```python
from build123d import *

# Parameters (mm, degrees)
CROQUIS1_R              = 2.1
CROQUIS1_R_2            = 3.4
SALIENTE_EXTRUIR1_DEPTH = 400


with BuildPart() as part:
    # Croquis1 → Saliente-Extruir1 (new body)
    with BuildSketch(Plane(origin=(0, 0, -50), x_dir=(-1, 0, 0), z_dir=(0, 0, -1))):
        with BuildLine():
            Line((14.7, -5.1), (14.3, -5.1))
            ThreePointArc((14.3, -5.1), (14.087867966, -5.012132034), (14, -4.8))
            Line((14, -4.8), (14, -4.4))
            ThreePointArc((14, -4.4), (13.912132034, -4.187867966), (13.7, -4.1))
            Line((13.7, -4.1), (13.3, -4.1))
            ThreePointArc((13.3, -4.1), (13.087867966, -4.187867966), (13, -4.4))
            Line((13, -4.4), (13, -7.95))
            ThreePointArc((13, -7.95), (12.912132034, -8.162132034), (12.7, -8.25))
            Line((12.7, -8.25), (9.789264108, -8.25))
            ThreePointArc((9.789264108, -8.25), (9.674477865, -8.22717164), (9.577160832, -8.162160788))
            Line((9.577160832, -8.162160788), (5.887896723, -4.473896751))
            ThreePointArc((5.887896723, -4.473896751), (5.822843922, -4.376559778), (5.8, -4.261735963))
            Line((5.8, -4.261735963), (5.8, 4.260735931))
            ThreePointArc((5.8, 4.260735931), (5.82283614, 4.375540961), (5.887867966, 4.472867966))
            Line((5.887867966, 4.472867966), (9.577132034, 8.162132034))
            ThreePointArc((9.577132034, 8.162132034), (9.674459039, 8.22716386), (9.789264069, 8.25))
            Line((9.789264069, 8.25), (12.7, 8.25))
            ThreePointArc((12.7, 8.25), (12.912132034, 8.162132034), (13, 7.95))
            Line((13, 7.95), (13, 4.4))
            ThreePointArc((13, 4.4), (13.087867966, 4.187867966), (13.3, 4.1))
            Line((13.3, 4.1), (13.7, 4.1))
            ThreePointArc((13.7, 4.1), (13.912132034, 4.187867966), (14, 4.4))
            Line((14, 4.4), (14, 4.8))
            ThreePointArc((14, 4.8), (14.087867966, 5.012132034), (14.3, 5.1))
            Line((14.3, 5.1), (14.7, 5.1))
            ThreePointArc((14.7, 5.1), (14.912132034, 5.187867966), (15, 5.4))
            Line((15, 5.4), (15, 12.5))
            ThreePointArc((15, 12.5), (14.267766953, 14.267766953), (12.5, 15))
            Line((12.5, 15), (5.4, 15))
            ThreePointArc((5.4, 15), (5.187867966, 14.912132034), (5.1, 14.7))
            Line((5.1, 14.7), (5.1, 14.3))
            ThreePointArc((5.1, 14.3), (5.012132034, 14.087867966), (4.8, 14))
            Line((4.8, 14), (4.4, 14))
            ThreePointArc((4.4, 14), (4.187867966, 13.912132034), (4.1, 13.7))
            Line((4.1, 13.7), (4.1, 13.3))
            ThreePointArc((4.1, 13.3), (4.187867966, 13.087867966), (4.4, 13))
            Line((4.4, 13), (7.95, 13))
            ThreePointArc((7.95, 13), (8.162132034, 12.912132034), (8.25, 12.7))
            Line((8.25, 12.7), (8.25, 9.788264069))
            ThreePointArc((8.25, 9.788264069), (8.22716386, 9.673459039), (8.162132034, 9.576132034))
            Line((8.162132034, 9.576132034), (4.473867966, 5.887867966))
            ThreePointArc((4.473867966, 5.887867966), (4.376540961, 5.82283614), (4.261735931, 5.8))
            Line((4.261735931, 5.8), (-4.260735892, 5.8))
            ThreePointArc((-4.260735892, 5.8), (-4.375522135, 5.82282836), (-4.472839168, 5.887839212))
            Line((-4.472839168, 5.887839212), (-8.162103277, 9.576103249))
            ThreePointArc((-8.162103277, 9.576103249), (-8.227156078, 9.673440222), (-8.25, 9.788264037))
            Line((-8.25, 9.788264037), (-8.25, 12.7))
            ThreePointArc((-8.25, 12.7), (-8.162132034, 12.912132034), (-7.95, 13))
            Line((-7.95, 13), (-4.4, 13))
            ThreePointArc((-4.4, 13), (-4.187867966, 13.087867966), (-4.1, 13.3))
            Line((-4.1, 13.3), (-4.1, 13.7))
            ThreePointArc((-4.1, 13.7), (-4.187867966, 13.912132034), (-4.4, 14))
            Line((-4.4, 14), (-4.8, 14))
            ThreePointArc((-4.8, 14), (-5.012132034, 14.087867966), (-5.1, 14.3))
            Line((-5.1, 14.3), (-5.1, 14.7))
            ThreePointArc((-5.1, 14.7), (-5.187867966, 14.912132034), (-5.4, 15))
            Line((-5.4, 15), (-12.5, 15))
            ThreePointArc((-12.5, 15), (-14.267766953, 14.267766953), (-15, 12.5))
            Line((-15, 12.5), (-15, 5.4))
            ThreePointArc((-15, 5.4), (-14.912132034, 5.187867966), (-14.7, 5.1))
            Line((-14.7, 5.1), (-14.3, 5.1))
            ThreePointArc((-14.3, 5.1), (-14.087867966, 5.012132034), (-14, 4.8))
            Line((-14, 4.8), (-14, 4.4))
            ThreePointArc((-14, 4.4), (-13.912132034, 4.187867966), (-13.7, 4.1))
            Line((-13.7, 4.1), (-13.3, 4.1))
            ThreePointArc((-13.3, 4.1), (-13.087867966, 4.187867966), (-13, 4.4))
            Line((-13, 4.4), (-13, 7.95))
            ThreePointArc((-13, 7.95), (-12.912132034, 8.162132034), (-12.7, 8.25))
            Line((-12.7, 8.25), (-9.788264037, 8.25))
            ThreePointArc((-9.788264037, 8.25), (-9.673440222, 8.227156078), (-9.576103249, 8.162103277))
            Line((-9.576103249, 8.162103277), (-5.887839212, 4.472839168))
            ThreePointArc((-5.887839212, 4.472839168), (-5.82282836, 4.375522135), (-5.8, 4.260735892))
            Line((-5.8, 4.260735892), (-5.8, -4.261735931))
            ThreePointArc((-5.8, -4.261735931), (-5.82283614, -4.376540961), (-5.887867966, -4.473867966))
            Line((-5.887867966, -4.473867966), (-9.576132034, -8.162132034))
            ThreePointArc((-9.576132034, -8.162132034), (-9.673459039, -8.22716386), (-9.788264069, -8.25))
            Line((-9.788264069, -8.25), (-12.7, -8.25))
            ThreePointArc((-12.7, -8.25), (-12.912132034, -8.162132034), (-13, -7.95))
            Line((-13, -7.95), (-13, -4.4))
            ThreePointArc((-13, -4.4), (-13.087867966, -4.187867966), (-13.3, -4.1))
            Line((-13.3, -4.1), (-13.7, -4.1))
            ThreePointArc((-13.7, -4.1), (-13.912132034, -4.187867966), (-14, -4.4))
            Line((-14, -4.4), (-14, -4.8))
            ThreePointArc((-14, -4.8), (-14.087867966, -5.012132034), (-14.3, -5.1))
            Line((-14.3, -5.1), (-14.7, -5.1))
            ThreePointArc((-14.7, -5.1), (-14.912132034, -5.187867966), (-15, -5.4))
            Line((-15, -5.4), (-15, -12.5))
            ThreePointArc((-15, -12.5), (-14.267766953, -14.267766953), (-12.5, -15))
            Line((-12.5, -15), (-5.4, -15))
            ThreePointArc((-5.4, -15), (-5.187867966, -14.912132034), (-5.1, -14.7))
            Line((-5.1, -14.7), (-5.1, -14.3))
            ThreePointArc((-5.1, -14.3), (-5.012132034, -14.087867966), (-4.8, -14))
            Line((-4.8, -14), (-4.4, -14))
            ThreePointArc((-4.4, -14), (-4.187867966, -13.912132034), (-4.1, -13.7))
            Line((-4.1, -13.7), (-4.1, -13.3))
            ThreePointArc((-4.1, -13.3), (-4.187867966, -13.087867966), (-4.4, -13))
            Line((-4.4, -13), (-7.95, -13))
            ThreePointArc((-7.95, -13), (-8.162132034, -12.912132034), (-8.25, -12.7))
            Line((-8.25, -12.7), (-8.25, -9.789264069))
            ThreePointArc((-8.25, -9.789264069), (-8.22716386, -9.674459039), (-8.162132034, -9.577132034))
            Line((-8.162132034, -9.577132034), (-4.472867966, -5.887867966))
            ThreePointArc((-4.472867966, -5.887867966), (-4.375540961, -5.82283614), (-4.260735931, -5.8))
            Line((-4.260735931, -5.8), (4.261735963, -5.8))
            ThreePointArc((4.261735963, -5.8), (4.376559778, -5.822843922), (4.473896751, -5.887896723))
            Line((4.473896751, -5.887896723), (8.162160788, -9.577160832))
            ThreePointArc((8.162160788, -9.577160832), (8.22717164, -9.674477865), (8.25, -9.789264108))
            Line((8.25, -9.789264108), (8.25, -12.7))
            ThreePointArc((8.25, -12.7), (8.162132034, -12.912132034), (7.95, -13))
            Line((7.95, -13), (4.4, -13))
            ThreePointArc((4.4, -13), (4.187867966, -13.087867966), (4.1, -13.3))
            Line((4.1, -13.3), (4.1, -13.7))
            ThreePointArc((4.1, -13.7), (4.187867966, -13.912132034), (4.4, -14))
            Line((4.4, -14), (4.8, -14))
            ThreePointArc((4.8, -14), (5.012132034, -14.087867966), (5.1, -14.3))
            Line((5.1, -14.3), (5.1, -14.7))
            ThreePointArc((5.1, -14.7), (5.187867966, -14.912132034), (5.4, -15))
            Line((5.4, -15), (12.5, -15))
            ThreePointArc((12.5, -15), (14.267766953, -14.267766953), (15, -12.5))
            Line((15, -12.5), (15, -5.4))
            ThreePointArc((15, -5.4), (14.912132034, -5.187867966), (14.7, -5.1))
        make_face()
        with Locations((-11.7, 11.7)):
            Circle(CROQUIS1_R, mode=Mode.SUBTRACT)
        with Locations((-11.7, -11.7)):
            Circle(CROQUIS1_R, mode=Mode.SUBTRACT)
        Circle(CROQUIS1_R_2, mode=Mode.SUBTRACT)
        with Locations((11.7, 11.7)):
            Circle(CROQUIS1_R, mode=Mode.SUBTRACT)
        with Locations((11.7, -11.7)):
            Circle(CROQUIS1_R, mode=Mode.SUBTRACT)
    extrude(amount=-SALIENTE_EXTRUIR1_DEPTH)


solid = part.part
```
The listing builds one solid part. Answer for the finished solid, in the listing's coordinates (mm). Round coordinates to 2 decimals unless told otherwise and drop trailing zeros. Order: outer loops, then holes, each group sorted by start corner. A loop starts at its lowest first (then second) coordinate and runs counter-clockwise, first axis right, second up. Notation, with made-up numbers: (53.25, -30.75) -> (63.25, -30.75) arc R32 cw to (63.25, -3.75) -> close; hole circle Ø9 at (-31, -0.5). An arc over 180 degrees is marked (long way). Answer as CSV lines item,"result". Start each with the question number.
(1) Find the intervals of material crossed by probe 1 along Y at (x, z) = (11.7, 78); probe 2 along Y at (x, z) = (12.25, 224), in increasing order. Write a range as from..to.
(2) The part is cut by section A-A (x = 0). Determine the outline of the cut face in (y, z), then the cut area to 3 significant figures.
(3) For a pull along X with two mould halves and no side action, classify faces 1 (the face through (0, 4, -50)), 2 (the face through (-15, -9, 147)), 3 (the face through (0, 5.8, 147)) as +X half, -X half, draft (parallel to the pull), parting line (faces both ways), or undercut.
(4) Flat-ended cylindrical pins translate along their axes: pin 1 Ø8 at (x, y) = (-1.5, -6) entering from -Z; pin 2 Ø7 at (y, z) = (0.5, 59) entering from -X. Find the tip coordinate at first contact, or state that the pin passes through.
(5) The part is cut by section C-C (z = 122). Count the separate pieces of the cut face and the enclosed holes in it, then the cut area to 3 significant figures.
Evaluation:
1,probe 1,"-15..-13.8, -9.6..-8.25, 8.25..9.6, 13.8..15"
1,probe 2,"-15..-13.73, -9.67..-8.25, 8.25..9.67, 13.73..15"
2,outline,"(-5.8, -50) -> (-3.4, -50) -> (-3.4, 350) -> (-5.8, 350) -> close; (3.4, -50) -> (5.8, -50) -> (5.8, 350) -> (3.4, 350) -> close"
2,area,"1,920 mm²"
3,face 1,"draft"
3,face 2,"-X half"
3,face 3,"undercut"
4,pin 1,"z = -50"
4,pin 2,"x = -5.8"
5,separate pieces,"1"
5,enclosed holes,"5"
5,area,"314 mm²"
